```python
from build123d import *

# Parameters (mm, degrees)
SKETCH_1_R          = 2
EXTRUDE_1_DEPTH     = 5
SKETCH_7_W          = 8
SKETCH_7_H          = 8
SKETCH_6_W          = 8
SKETCH_6_H          = 8
SKETCH_9_W          = 8
SKETCH_9_H          = 8
EXTRUDE_5_DEPTH     = 10
SKETCH_1_6_R        = 2
CUT_EXTRUDE_2_DEPTH = 99
SKETCH_14_W         = 8
SKETCH_14_H         = 8
SKETCH_15_W         = 8
SKETCH_15_H         = 8
EXTRUDE_7_REACH     = 31
SKETCH_17_W         = 8
SKETCH_17_H         = 8
SKETCH_1_7_R        = 2
CUT_EXTRUDE_4_DEPTH = 33.5


with BuildPart() as part:
    # 草图1 → 凸台-拉伸1 (new body)
    with BuildSketch(Plane.XY):
        with BuildLine():
            Line((-15, 4), (-15, -4))
            Line((-15, -4), (0, -4))
            ThreePointArc((0, -4), (2.828427125, -2.828427125), (4, 0))
            Line((4, 0), (4, 15))
            Line((4, 15), (-4, 15))
            Line((-4, 15), (-4, 8))
            ThreePointArc((-4, 8), (-5.171572875, 5.171572875), (-8, 4))
            Line((-8, 4), (-15, 4))
        make_face()
        Circle(SKETCH_1_R, mode=Mode.SUBTRACT)
    extrude(amount=EXTRUDE_1_DEPTH)

    # 草图7 → 放样2 section 0
    with BuildSketch(Plane.XY.offset(5)):
        with Locations((-13, 0)):
            Rectangle(SKETCH_7_W, SKETCH_7_H)
    # 草图6 → 放样2 section 1
    with BuildSketch(Plane.XY.offset(38)):
        with Locations((-11, 0)):
            Rectangle(SKETCH_6_W, SKETCH_6_H)
    loft()

    # 草图9 → 凸台-拉伸5 (add)
    with BuildSketch(Plane(origin=(-25, 0, 0), x_dir=(0, 0, -1), z_dir=(1, 0, 0))):
        with Locations((-34, 0)):
            Rectangle(SKETCH_9_W, SKETCH_9_H)
    extrude(amount=EXTRUDE_5_DEPTH)

    # 草图1<6> → 切除-拉伸2 (cut)
    with BuildSketch(Plane.XY):
        with Locations((-20, 0)):
            Circle(SKETCH_1_6_R)
    extrude(amount=CUT_EXTRUDE_2_DEPTH, mode=Mode.SUBTRACT)

    # 草图14 → 放样3 section 0
    with BuildSketch(Plane.XY):
        with Locations((0, 11)):
            Rectangle(SKETCH_14_W, SKETCH_14_H)
    # 草图15 → 放样3 section 1
    with BuildSketch(Plane.XY.offset(18)):
        with Locations((0, 19)):
            Rectangle(SKETCH_15_W, SKETCH_15_H)
    loft()

    # 凸台-拉伸7: up to this face of the body (flat: up to its plane)
    extrude_7_end = Plane(part.part.faces().sort_by_distance((0, 19, 9))[0])
    # 草图17 → 凸台-拉伸7 (add, up to the picked face)
    with BuildSketch(Plane(origin=(0, 25, 0), x_dir=(1, 0, 0), z_dir=(0, 1, 0)), mode=Mode.PRIVATE) as extrude_7_sk1:
        with Locations((0, -14)):
            Rectangle(SKETCH_17_W, SKETCH_17_H)
    extrude_7_tool1 = split(extrude(extrude_7_sk1.sketch, amount=-EXTRUDE_7_REACH, mode=Mode.PRIVATE), bisect_by=extrude_7_end, keep=Keep.BOTH, mode=Mode.PRIVATE)
    add(extrude_7_tool1.solids().sort_by_distance((0, 25, 14))[0])

    # 草图1<7> → 切除-拉伸4 (cut)
    with BuildSketch(Plane.XY):
        with Locations((0, 20)):
            Circle(SKETCH_1_7_R)
    extrude(amount=CUT_EXTRUDE_4_DEPTH, mode=Mode.SUBTRACT)


solid = part.part
```
Check sheet for the modelled part. Datum: model origin and axes. Units: mm. A direction names the side the tool comes from. Give positions to 0.01 mm unless a question says otherwise; leave off trailing zeros. Loops run counter-clockwise (first coordinate to the right, second up) from the corner with the lowest first, then second, coordinate; pieces in that order, holes last. Notation, with made-up numbers: M 55.25,-34 L 113.25,-34 A4 cw 113.25,-29 Z; hole C 58.5,-2 d1. An arc over 180 degrees is marked long. Answer as CSV lines item,"result".
Item 1: Sectioned sample at A-A, the plane y = 20. Enter the section's corners in (x, z), then the cut area to 3 significant figures.
Reply:
outline,"M -4,10 L -2,10 L -2,18 L -4,18 Z; M 2,10 L 4,10 L 4,18 L 2,18 Z"
area,"32.0 mm^2"
Item 2: Draft check along Y on faces 4 (the face through (0, 18, 14)), 5 (the face through (-0.06, 12.15, 11.59)), 6 (the face through (-16, 0, 5)). Enter one of: pulls with the +Y half, pulls with the -Y half, needs draft (parallel to the pull), parting line crosses it, or undercut.
Reply:
face 4,"undercut"
face 5,"pulls with the -Y half"
face 6,"needs draft"
Item 3: Sectioned sample at C-C, the plane z = 15.5. Enter the section's corners in (x, y), then the cut area to 3 significant figures.
Reply:
outline,"M -16.36,-4 L -8.36,-4 L -8.36,4 L -16.36,4 Z; M -4,13.89 L 4,13.89 L 4,25 L -4,25 Z; hole C 0,20 d4"
area,"140 mm^2"
Item 4: Depth check by flat-ended pin: pin 1 Ø1.5 at (y, z) = (0, 32.5) entering from +X; pin 2 Ø14.5 at (x, z) = (-13.5, 22) entering from +Y; pin 3 Ø1.5 at (x, z) = (-2.5, 8.5) entering from -Y; pin 4 Ø12 at (y, z) = (20, 7.5) entering from +X. Enter the tip coordinate at first touch or a pass-through.
Reply:
pin 1,"x = -7.29"
pin 2,"y = 4"
pin 3,"y = 10.44"
pin 4,"x = 4"
Item 5: Set-up check for faces 1 (the face through (-16.23, 0.06, 17.68)), 2 (the face through (-15, 0, 2)), 3 (the face through (-4, 17, 9)): record each of +Z, -Z, +X, -X, +Y, -Y from which the full face is reachable in a straight line by a thin tool's end or side.
Reply:
face 1,"-X, +Y, -Y"
face 2,"-Z, -X, +Y, -Y"
face 3,"+Z, -Z, -X, +Y"
Item 6: Sectioned sample at D-D, the plane x = -11.25. Enter the section's corners in (y, z), then the cut area to 3 significant figures.
Reply:
outline,"M -4,0 L 4,0 L 4,38 L -4,38 Z"
area,"304 mm^2"
Item 7: Scan lines: L1, parallel to Y at x = -20, z = 32; L2, parallel to X at y = 0, z = 35.75. Record each from-to range of solid material in increasing order.
Reply:
L1,"-4 to -2, 2 to 4"
L2,"-25 to -22, -18 to -7.14"
Item 8: Sectioned sample at B-B, the plane x = -20. Enter the section's corners in (y, z).
Reply:
outline,"M -4,30 L -2,30 L -2,38 L -4,38 Z; M 2,30 L 4,30 L 4,38 L 2,38 Z"
